```python
from build123d import *

# Parameters (mm, degrees)
F0_R     = 4.5
F1_DEPTH = 25
F3_DEPTH = 50
F5_DEPTH = 50
F6_R     = 4.5
F7_DEPTH = 17
F8_R     = 4.5
F9_DEPTH = 17


with BuildPart() as f1:
    # F0 (on Right) → F1 (new body, symmetric)
    with BuildSketch(Plane.YZ):
        with BuildLine():
            Line((0, 7), (0, 0))
            Line((0, 0), (-13.5, 0))
            Line((-13.5, 0), (-45.723576, -45.306083))
            ThreePointArc((-45.723576, -45.306083), (-48.401067, -55.719942), (-43.421567, -65.25))
            Line((-43.421567, -65.25), (-33.5, -74))
            Line((-33.5, -74), (-13.5, -74))
            Line((-13.5, -74), (3, -74))
            Line((3, -74), (3, -71))
            Line((3, -71), (0, -71))
            Line((0, -71), (0, -72))
            Line((0, -72), (-5.5, -72))
            Line((-5.5, -72), (-5.5, -5))
            Line((-5.5, -5), (4.5, -5))
            Line((4.5, -5), (4.5, 7))
            Line((4.5, 7), (0, 7))
        make_face()
        with Locations((-33.5, -54)):
            Circle(F0_R, mode=Mode.SUBTRACT)
    extrude(amount=F1_DEPTH, both=True)

    # F2 (on face) → F3 (cut, through all)
    with BuildSketch(Plane.YZ.offset(25)):
        Polygon((4.5, 7), (2.2, 7), (4.5, -0.822673), align=None)
    extrude(amount=-F3_DEPTH, mode=Mode.SUBTRACT)

    # F4 (on face) → F5 (cut, through all)
    with BuildSketch(Plane.YZ.offset(25)):
        Polygon((0, -71), (0, -72), (1.5, -71), align=None)
        Polygon((3, -71), (1.5, -71), (3, -72), align=None)
    extrude(amount=-F5_DEPTH, mode=Mode.SUBTRACT)

    # F6 (on face) → F7 (cut)
    with BuildSketch(Plane.YZ.offset(25)):
        with BuildLine():
            Line((-13.5, -74), (-13.5, 0))
            Line((-13.5, 0), (-45.723576, -45.306083))
            ThreePointArc((-45.723576, -45.306083), (-48.401067, -55.719942), (-43.421567, -65.25))
            Line((-43.421567, -65.25), (-33.5, -74))
            Line((-33.5, -74), (-13.5, -74))
        make_face()
        with Locations((-33.5, -54)):
            Circle(F6_R, mode=Mode.SUBTRACT)
    extrude(amount=-F7_DEPTH, mode=Mode.SUBTRACT)

    # F8 (on face) → F9 (cut)
    with BuildSketch(Plane(origin=(-25, 0, 0), x_dir=(0, -1, 0), z_dir=(-1, 0, 0))):
        with BuildLine():
            Line((45.723576, -45.306083), (13.5, 0))
            Line((13.5, 0), (13.5, -74))
            Line((13.5, -74), (33.5, -74))
            Line((33.5, -74), (43.421567, -65.25))
            ThreePointArc((43.421567, -65.25), (48.401067, -55.719942), (45.723576, -45.306083))
        make_face()
        with Locations((33.5, -54)):
            Circle(F8_R, mode=Mode.SUBTRACT)
    extrude(amount=-F9_DEPTH, mode=Mode.SUBTRACT)


solid = f1.part
```
Geometry: final body of the model. Coordinates: model frame, mm. A direction names the side the tool comes from. Give positions to 0.01 mm unless a question says otherwise; leave off trailing zeros. Loops run counter-clockwise (first coordinate to the right, second up) from the corner with the lowest first, then second, coordinate; pieces in that order, holes last. Notation, with made-up numbers: (77, 16) -> (124, 16) arc R21 ccw to (124, 47) -> close; hole circle Ø8 at (30, -1). An arc over 180 degrees is marked (long way). Use one line per item in the form item = value.
Item 1: Section query D-D on z = -15.5. Output: boundary loops of the cut face in (x, y).
A:
outline = (-25, -13.5) -> (-8, -13.5) -> (-8, -24.52) -> (8, -24.52) -> (8, -13.5) -> (25, -13.5) -> (25, -5.5) -> (-25, -5.5) -> close
Item 2: Pin query (flat end, axial travel): P1, Ø1.5, axis at y = -15.5, z = -54, coming from the -X side; P2, Ø10, axis at x = 4, y = -11.5, coming from the +Z side; P3, Ø2, axis at x = 3.5, z = -73, coming from the +Y side. Return the tip coordinate at first contact, or that it passes through.
A:
P1 = -8
P2 = 0
P3 = 3
Item 3: Section query B-B on x = 2. Output: boundary loops of the cut face in (y, z).
A:
outline = (-45.72, -45.31) arc R15 ccw to (-43.42, -65.25) -> (-33.5, -74) -> (3, -74) -> (3, -72) -> (1.5, -71) -> (0, -72) -> (-5.5, -72) -> (-5.5, -5) -> (4.5, -5) -> (4.5, -0.82) -> (2.2, 7) -> (0, 7) -> (0, 0) -> (-13.5, 0) -> close; hole circle Ø9 at (-33.5, -54)
Item 4: Draft query along Z for faces 1 (the face through (0, -3, -72)), 2 (the face through (0, -1, -5)), 3 (the face through (0, 0, 4)), 4 (the face through (0, 1, 7)). Return one class per face: pulls with the +Z half, pulls with the -Z half, needs draft (parallel to the pull), parting line crosses it, or undercut.
A:
face_1 = undercut
face_2 = undercut
face_3 = needs draft
face_4 = pulls with the +Z half
Item 5: Access query for faces 5 (the face through (17, -13.5, -38)), 6 (the face through (0, -7, 0)), 7 (the face through (0, 3, -73)), 8 (the face through (-8, -27, -45)), 9 (the face through (0, 4.5, -3)). Directions: +Z, -Z, +X, -X, +Y, -Y. A direction counts if a zero-diameter tool reaches every point of the face in a straight line with its end or side. Return the directions, or none.
A:
face_5 = +Z, -Z, +X, -Y
face_6 = +Z, +X, -X, -Y
face_7 = -Z, +X, -X, +Y
face_8 = +Z, -Z, -X, -Y
face_9 = +Z, -Z, +X, -X, +Y
Item 6: Section query A-A on z = -54. Output: boundary loops of the cut face in (x, y).
A:
outline = (-25, -13.5) -> (-8, -13.5) -> (-8, -29) -> (8, -29) -> (8, -13.5) -> (25, -13.5) -> (25, -5.5) -> (-25, -5.5) -> close; (-8, -48.5) -> (8, -48.5) -> (8, -38) -> (-8, -38) -> close
Item 7: Section query C-C on x = 20.5. Output: boundary loops of the cut face in (y, z), and give its area (3 significant figures).
A:
outline = (-13.5, -74) -> (3, -74) -> (3, -72) -> (1.5, -71) -> (0, -72) -> (-5.5, -72) -> (-5.5, -5) -> (4.5, -5) -> (4.5, -0.82) -> (2.2, 7) -> (0, 7) -> (0, 0) -> (-13.5, 0) -> close
area = 683 mm^2
Item 8: Line query: probe 1 along Z at (x, y) = (15.5, -5); probe 2 along Y at (x, z) = (20.5, -7); probe 3 along Y at (x, z) = (5.5, -57). Output: solid intervals per line, ascending.
A:
probe_1 = -74 to -72, -5 to 0
probe_2 = -13.5 to -5.5
probe_3 = -48.2 to -36.85, -30.15 to -5.5
